Here's how the part is built. I have some questions about the finished solid (model axes, mm). A direction names the side the tool comes from. Coordinates: 2 decimals unless noted, no trailing zeros. Loops run counter-clockwise (first coordinate to the right, second up) from the corner with the lowest first, then second, coordinate; pieces in that order, holes last. Notation, with made-up numbers: (-1, -2) -> (12, -2) arc R25 ccw to (12, 24) -> close; hole circle Ø8 at (-24, -27.75). An arc over 180 degrees is marked (long way). Answer as a JSON object with one key per item and string values. Group by question number.
1) I want a section at A-A (z = 0). Write out the boundary of the cut face in (x, y), then the cut area to 3 significant figures.
2) I want a section at B-B (x = 0). Count the separate pieces of the cut face and the enclosed holes in it, then the cut area to 3 significant figures.
3) I'm going to push flat-ended pins straight in: pin 1 (1.2 mm diameter, centred on y = 7, z = -10, fed in from +X); pin 2 (8 mm diameter, centred on y = 15.5, z = -14.5, fed in from -X); pin 3 (10 mm diameter, centred on y = 15.5, z = -5, fed in from +X); pin 4 (5.5 mm diameter, centred on x = -0.5, y = 9, fed in from +Z). Where does each tip first touch, or does it pass through?
4) Which directions (+Z, -Z, +X, -X, +Y, -Y) give clear straight access to the entire face, cutting with the end or side of a thin tool? Please do faces 1 (the flat face through (-3.987, 4, 10)), 2 (the flat face through (12.202, 3, 0)).
5) If we mould it in two halves opening along X, with no side actions, what happens to faces 3 (the flat face through (-7.497, 2.79, -11.033)), 4 (the cylindrical face through (19.334, 3.241, -2.539))? For each: +X half, -X half, draft (parallel to the pull), parting line (faces both ways), or undercut.
6) I need wall thicknesses on probe 1 along X at (y, z) = (10, 0); probe 2 along Z at (x, y) = (-11, -4.5); probe 3 along X at (y, z) = (19.5, -7). Which ranges of each line are inside material? Lowest first, please. Write a range as [from, to].
```python
from build123d import *

# Parameters (mm, degrees)
SKETCH1_R           = 17
BOSS_EXTRUDE1_DEPTH = 3
SKETCH3_R           = 17
BOSS_EXTRUDE2_DEPTH = 3
BOSS_EXTRUDE3_DEPTH = 31
SKETCH7_R           = 1.751351815
CUT_EXTRUDE11_DEPTH = 50
CUT_EXTRUDE1_DEPTH  = 50
SKETCH8_W           = 7.5
SKETCH8_H           = 2.5
CUT_EXTRUDE12_DEPTH = 40
SKETCH9_R           = 19.5
SKETCH9_R_2         = 18
BOSS_EXTRUDE4_DEPTH = 37
FILLET1_R           = 3
SKETCH10_R          = 17
SKETCH10_R_2        = 16.5
CUT_EXTRUDE13_DEPTH = 3
SKETCH11_R          = 19.5
BOSS_EXTRUDE5_DEPTH = 3


with BuildPart() as part:
    # Sketch1 → Boss-Extrude1 (new body)
    with BuildSketch(Plane(origin=(0, -15, 0), x_dir=(1, 0, 0), z_dir=(0, 1, 0))):
        with Locations(Location((0, 0, 0), (0, 0, 270))):
            Circle(SKETCH1_R)
    extrude(amount=BOSS_EXTRUDE1_DEPTH)



with BuildPart() as body_2:
    # Sketch3 → Boss-Extrude2 (new body)
    with BuildSketch(Plane(origin=(0, 21, 0), x_dir=(1, 0, 0), z_dir=(0, 1, 0))):
        with Locations(Location((0, 0, 0), (0, 0, 270))):
            Circle(SKETCH3_R)
    extrude(amount=-BOSS_EXTRUDE2_DEPTH)


with BuildPart() as part_1:
    add(part.part)

    add(body_2.part)  # Boss-Extrude3 merges body 2
    # Sketch6 → Boss-Extrude3 (add)
    with BuildSketch(Plane(origin=(0, -12, 0), x_dir=(1, 0, 0), z_dir=(0, 1, 0))):
        Polygon((-10.39609313, -6.860559341), (-11.68775931, -8.152225055), (-12.244775891, -7.288892753), (-12.738139369, -6.387668662), (-13.165283017, -5.453239195), (-13.523988426, -4.490460269), (-13.812389225, -3.504338907), (-14.028987847, -2.499999944), (-12.202296406, -2.499999944), (-12.202296406, 2.499999944), (-14.028987847, 2.499999944), (-13.812389225, 3.504338907), (-13.523988426, 4.490460269), (-13.165283017, 5.453239195), (-12.738139369, 6.387668662), (-12.244775891, 7.288892753), (-11.68775931, 8.152225055), (-10.39609313, 6.860559341), (-6.860559341, 10.39609313), (-8.152225055, 11.68775931), (-7.288892753, 12.244775891), (-6.387668662, 12.738139369), (-5.453239195, 13.165283017), (-4.490460269, 13.523988426), (-3.504338907, 13.812389225), (-2.499999944, 14.028987847), (-2.499999944, 12.174172863), (2.499999944, 12.202296406), (2.499999944, 14.028987847), (3.504338907, 13.812389225), (4.490460269, 13.523988426), (5.453239195, 13.165283017), (6.387668662, 12.738139369), (7.288892753, 12.244775891), (8.152225055, 11.68775931), (6.860559341, 10.39609313), (10.39609313, 6.860559341), (11.68775931, 8.152225055), (12.244775891, 7.288892753), (12.738139369, 6.387668662), (13.165283017, 5.453239195), (13.523988426, 4.490460269), (13.812389225, 3.504338907), (14.028987847, 2.499999944), (12.202296406, 2.499999944), (12.202296406, -2.499999944), (14.028987847, -2.499999944), (13.812389225, -3.504338907), (13.523988426, -4.490460269), (13.165283017, -5.453239195), (12.738139369, -6.387668662), (12.244775891, -7.288892753), (11.68775931, -8.152225055), (10.39609313, -6.860559341), (6.860559341, -10.39609313), (8.152225055, -11.68775931), (7.288892753, -12.244775891), (6.387668662, -12.738139369), (5.453239195, -13.165283017), (4.490460269, -13.523988426), (3.504338907, -13.812389225), (2.499999944, -14.028987847), (2.499999944, -12.202296406), (-2.499999944, -12.202296406), (-2.499999944, -14.028987847), (-3.504338907, -13.812389225), (-4.490460269, -13.523988426), (-5.453239195, -13.165283017), (-6.387668662, -12.738139369), (-7.288892753, -12.244775891), (-8.152225055, -11.68775931), (-6.860559341, -10.39609313), align=None)
    extrude(amount=BOSS_EXTRUDE3_DEPTH)

    # Sketch7 → Cut-Extrude11 (cut)
    with BuildSketch(Plane(origin=(-0.068553102, 0, -12.187849043), x_dir=(-0.9999841817006155, 0, 0.005624619858302935), z_dir=(-0.005624619858302935, 0, -0.9999841817006155))):
        with Locations((-0.120761258, 16)):
            Circle(SKETCH7_R)
    extrude(amount=-CUT_EXTRUDE11_DEPTH, mode=Mode.SUBTRACT)

    # Sketch2 → Cut-Extrude1 (cut)
    with BuildSketch(Plane(origin=(0, -15, 0), x_dir=(1, 0, 0), z_dir=(0, 1, 0))):
        with BuildLine():
            Line((1.514793699, 1.566442938), (-1.521232282, 1.566442938))
            ThreePointArc((-1.521232282, 1.566442938), (-0.003219291, -2.164389177), (1.514793699, 1.566442938))
        make_face()
    extrude(amount=CUT_EXTRUDE1_DEPTH, mode=Mode.SUBTRACT)

    # Sketch8 → Cut-Extrude12 (cut)
    with BuildSketch(Plane(origin=(0, -15, 0), x_dir=(1, 0, 0), z_dir=(0, 1, 0))):
        with Locations((-0.237061367, 10.255385433)):
            Rectangle(SKETCH8_W, SKETCH8_H)
    cut_extrude12 = extrude(amount=CUT_EXTRUDE12_DEPTH, mode=Mode.SUBTRACT)

    # Mirror1: Cut-Extrude12 across plane
    add(cut_extrude12.mirror(Plane.XY), mode=Mode.SUBTRACT)

    # Sketch10 → Cut-Extrude13 (cut)
    with BuildSketch(Plane(origin=(0, 21, 0), x_dir=(1, 0, 0), z_dir=(0, 1, 0))):
        with Locations(Location((0, 0, 0), (0, 0, 270))):
            Circle(SKETCH10_R)
        with Locations(Location((0, 0, 0), (0, 0, 270))):
            Circle(SKETCH10_R_2, mode=Mode.SUBTRACT)
    extrude(amount=-CUT_EXTRUDE13_DEPTH, mode=Mode.SUBTRACT)



with BuildPart() as body_2_2:
    # Sketch9 → Boss-Extrude4 (new body)
    with BuildSketch(Plane(origin=(0, -15, 0), x_dir=(1, 0, 0), z_dir=(0, 1, 0))):
        with Locations(Location((0, 0, 0), (0, 0, 270))):
            Circle(SKETCH9_R)
        with Locations(Location((0, 0, 0), (0, 0, 270))):
            Circle(SKETCH9_R_2, mode=Mode.SUBTRACT)
    extrude(amount=BOSS_EXTRUDE4_DEPTH)

    # Fillet1
    # the kernel refuses this fillet: 3 mm, written as the material it takes off along each edge
    with BuildSketch(Plane(origin=(0, 22, 0), x_dir=(0, 0, 1), z_dir=(-1, 0, 0))) as fillet1_piece_1:
        with BuildLine():
            CenterArc((21, -2.598076211), FILLET1_R, 120, 60)
            Line((19.5, 0), (19.47, 0.051961524))
            ThreePointArc((19.47, 0.051961524), (18.75, 0.06), (18, 0.06))
            Line((18, 0.06), (17.94, 0))
            Line((17.94, 0), (17.94, -2.598076211))
            Line((17.94, -2.598076211), (18, -2.598076211))
        make_face()
    revolve(axis=Axis((0, 22, 0), (0, 1, 0)), mode=Mode.SUBTRACT)


with BuildPart() as part_2:
    add(part_1.part)

    add(body_2_2.part)  # Boss-Extrude5 merges body 2 2
    # Sketch11 → Boss-Extrude5 (add)
    with BuildSketch(Plane(origin=(0, -15, 0), x_dir=(1, 0, 0), z_dir=(0, 1, 0))):
        with Locations(Location((0, 0, 0), (0, 0, 270))):
            Circle(SKETCH11_R)
    extrude(amount=BOSS_EXTRUDE5_DEPTH)


solid = part_2.part
```
Determined:
{
 "1": {"outline": "(-19.5, -15) -> (19.5, -15) -> (19.5, 22) arc R3 ccw to (18, 19.4) -> (18, -12) -> (12.2, -12) -> (12.2, 18) -> (16.5, 18) -> (16.5, 21) -> (2.17, 21) -> (2.17, -12) -> (-2.18, -12) -> (-2.18, 21) -> (-16.5, 21) -> (-16.5, 18) -> (-12.2, 18) -> (-12.2, -12) -> (-18, -12) -> (-18, 19.4) arc R3 ccw to (-19.5, 22) -> close", "area": "904 mm^2"},
 "2": {"separate pieces": "5", "enclosed holes": "0", "area": "705 mm^2"},
 "3": {"pin 1": "x = 17.08", "pin 2": "x = -16.43", "pin 3": "x = 19.5", "pin 4": "z = 19.5"},
 "4": {"face 1": "+Y", "face 2": "none"},
 "5": {"face 3": "undercut", "face 4": "parting line"},
 "6": {"probe 1": "[-19.5, -18], [-12.2, -2.18], [2.17, 12.2], [18, 19.5]", "probe 2": "[-16.1, -14.25], [-7.46, 7.46], [14.25, 16.1]", "probe 3": "[-18.2, -16.58], [-14.94, 14.94], [16.58, 18.2]"}
}
